Work out the finished part from the listing and answer in its coordinate system (mm). Face numbers are marked on the shaded views. A direction names the side the tool comes from. Round coordinates to 2 decimals unless told otherwise and drop trailing zeros. Loops run counter-clockwise (first coordinate to the right, second up) from the corner with the lowest first, then second, coordinate; pieces in that order, holes last.
```python
from build123d import *

# Parameters (mm, degrees)
SKETCH_1_R               = 37.5
SKETCH_1_R_2             = 34.5
EXTRUDE_1_DEPTH          = 24.5
SKETCH_2_R               = 1.5
EXTRUDE_2_DEPTH          = 5
PATTERN_CIRCULAR_1_COUNT = 6
SKETCH_3_R               = 37.5
SKETCH_3_R_2             = 19
EXTRUDE_3_DEPTH          = 3
SKETCH_4_R               = 1
CUT_EXTRUDE_1_DEPTH      = 3
CUT_EXTRUDE_START        = -21
CUT_EXTRUDE_2_DEPTH      = 21
PATTERN_CIRCULAR_2_COUNT = 4


with BuildPart() as part:
    # Эскиз1 → Бобышка-Вытянуть1 (new body)
    with BuildSketch(Plane.XY):
        Circle(SKETCH_1_R)
        Circle(SKETCH_1_R_2, mode=Mode.SUBTRACT)
    extrude(amount=EXTRUDE_1_DEPTH)

    # Эскиз2 → Бобышка-Вытянуть2 (add)
    with BuildSketch(Plane(origin=(0, 0, 0), x_dir=(-1, 0, 0), z_dir=(0, 0, -1))):
        with BuildLine():
            Line((-3.69551813, 42.530733729), (-5.977950182, 37.020455313))
            ThreePointArc((-5.977950182, 37.020455313), (0, 37.5), (5.977950182, 37.020455313))
            Line((5.977950182, 37.020455313), (3.69551813, 42.530733729))
            ThreePointArc((3.69551813, 42.530733729), (0, 45), (-3.69551813, 42.530733729))
        make_face()
        with Locations((0, 41)):
            Circle(SKETCH_2_R, mode=Mode.SUBTRACT)
    extrude_2 = extrude(amount=-EXTRUDE_2_DEPTH)

    # Круговой массив1: Бобышка-Вытянуть2 ×6 about axis
    pattern_circular_1_axis = Axis((0, 0, 0), (0, 0, 1))
    for i in range(1, PATTERN_CIRCULAR_1_COUNT):
        add(extrude_2.rotate(pattern_circular_1_axis, i * 360 / PATTERN_CIRCULAR_1_COUNT))

    # Эскиз3 → Бобышка-Вытянуть3 (add)
    with BuildSketch(Plane.XY.offset(24.5)):
        with Locations(Location((0, 0, 0), (0, 0, 159.172768539))):
            Circle(SKETCH_3_R)
        Circle(SKETCH_3_R_2, mode=Mode.SUBTRACT)
    extrude(amount=EXTRUDE_3_DEPTH)

    # Эскиз4 → Вырез-Вытянуть1 (cut)
    with BuildSketch(Plane.XY.offset(27.5)):
        with Locations((22, 0)):
            Circle(SKETCH_4_R)
        with Locations((0, -22)):
            Circle(SKETCH_4_R)
        with Locations((-22, 0)):
            Circle(SKETCH_4_R)
        with Locations((0, 22)):
            Circle(SKETCH_4_R)
    extrude(amount=-CUT_EXTRUDE_1_DEPTH, mode=Mode.SUBTRACT)

    # Эскиз5 → Вырез-Вытянуть2 (cut)
    with BuildSketch(Plane.XY.offset(27.5).offset(CUT_EXTRUDE_START)):
        with BuildLine():
            Line((0, 0), (34.645482469, 14.350628714))
            ThreePointArc((34.645482469, 14.350628714), (26.516504294, 26.516504294), (14.350628714, 34.645482469))
            Line((14.350628714, 34.645482469), (0, 0))
        make_face()
    cut_extrude_2 = extrude(amount=CUT_EXTRUDE_2_DEPTH, mode=Mode.SUBTRACT)

    # Круговой массив2: Вырез-Вытянуть2 ×4 about axis
    pattern_circular_2_axis = Axis((0, 0, 24.5), (0, 0, -1))
    for i in range(1, PATTERN_CIRCULAR_2_COUNT):
        add(cut_extrude_2.rotate(pattern_circular_2_axis, i * 360 / PATTERN_CIRCULAR_2_COUNT), mode=Mode.SUBTRACT)


solid = part.part
```
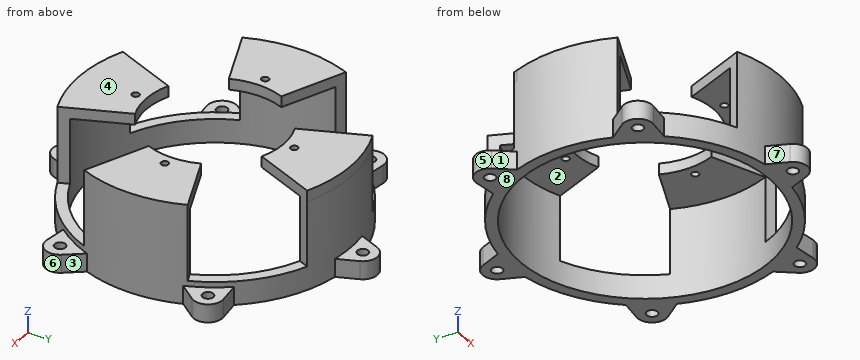
1. Find section B-B (y = 41). Write down the section's boundary in (x, z).
Answer key:
outline: (-4.33, 0) - (-1.5, 0) - (-1.5, 5) - (-4.33, 5) - close; (1.5, 0) - (4.33, 0) - (4.33, 5) - (1.5, 5) - close
2. Find section D-D (x = 24). Write down the section's boundary in (y, z).
Answer key:
outline: (-28.81, 0) - (-24.78, 0) - (-24.78, 6.5) - (-28.81, 6.5) - close; (-9.94, 24.5) - (9.94, 24.5) - (9.94, 27.5) - (-9.94, 27.5) - close; (24.78, 0) - (28.81, 0) - (28.81, 6.5) - (24.78, 6.5) - close
3. Determine the mould class of the marked faces 5, 6, 7 and 8 for opening direction Y: +Y half, -Y half, draft (parallel to the pull), parting line (faces both ways), or undercut.
Answer key:
face 5: undercut
face 6: undercut
face 7: -Y half
face 8: draft
4. Consider probe 1 along Y at (x, z) = (0, 1.55); probe 2 along Y at (x, z) = (0, 19.5); probe 3 along Z at (x, y) = (-22.5, -27.5). Determine where each line is inside the solid, lowest interval first.
Answer key:
probe 1: y = -45 to -42.5, -39.5 to -34.5, 34.5 to 39.5, 42.5 to 45
probe 2: y = -37.5 to -34.5, 34.5 to 37.5
probe 3: z = 0 to 6.5
5. Which of the six approach directions +Z, -Z, +X, -X, +Y, -Y give full straight-line access (tool end or side, diameter ignored) to the marked faces 1, 2, 3 and 4?
Answer key:
face 1: +Z, -Z, -X
face 2: -Z
face 3: +Z, -Z, +X
face 4: +Z, +X, -X, +Y, -Y
6. Given pin 1 (6 mm diameter, centred on y = 7.5, z = 20, fed in from -X); pin 2 (5 mm diameter, centred on x = 3.5, y = 22.5, fed in from -Z); pin 3 (5 mm diameter, centred on x = -34.5, y = -18.5, fed in from +Z); pin 4 (6.5 mm diameter, centred on x = -22.5, y = 18.5, fed in from +Z), each flat-ended and moving along its own axis, determine where each tip first touches the part or whether it passes through.
Answer key:
pin 1: stops at x = -37.23
pin 2: stops at z = 24.5
pin 3: stops at z = 6.5
pin 4: passes through
7. Find section C-C (z = 16.5). Write down the section's boundary in (x, y), then the cut area to 3 significant figures.
Answer key:
outline: (-34.65, -14.35) - (-31.87, -13.2) arc R34.5 cw to (-31.87, 13.2) - (-34.65, 14.35) arc R37.5 ccw to start; (-14.35, -34.65) arc R37.5 ccw to (14.35, -34.65) - (13.2, -31.87) arc R34.5 cw to (-13.2, -31.87) - close; (-14.35, 34.65) - (-13.2, 31.87) arc R34.5 cw to (13.2, 31.87) - (14.35, 34.65) arc R37.5 ccw to start; (31.87, -13.2) - (34.65, -14.35) arc R37.5 ccw to (34.65, 14.35) - (31.87, 13.2) arc R34.5 cw to start
area: 339 mm2
8. Find section A-A (z = 25.75). Write down the section's boundary in (x, y).
Answer key:
outline: (-34.65, -14.35) - (-17.55, -7.27) arc R19 cw to (-17.55, 7.27) - (-34.65, 14.35) arc R37.5 ccw to start; (-14.35, -34.65) arc R37.5 ccw to (14.35, -34.65) - (7.27, -17.55) arc R19 cw to (-7.27, -17.55) - close; (-14.35, 34.65) - (-7.27, 17.55) arc R19 cw to (7.27, 17.55) - (14.35, 34.65) arc R37.5 ccw to start; (17.55, -7.27) - (34.65, -14.35) arc R37.5 ccw to (34.65, 14.35) - (17.55, 7.27) arc R19 cw to start; hole circle Ø2 at (-22, 0); hole circle Ø2 at (0, -22); hole circle Ø2 at (0, 22); hole circle Ø2 at (22, 0)
